```python
from build123d import *

# Parameters (mm, degrees)
BOSS_EXTRUDE1_DEPTH = 10
SKETCH6_W           = 35.294117648
SKETCH6_H           = 18.823529412
BOSS_EXTRUDE3_DEPTH = 500
SKETCH8_W           = 35.294117648
SKETCH8_H           = 20.234009988
BOSS_EXTRUDE4_DEPTH = 50
SKETCH9_W           = 699.8
SKETCH9_H           = 322.2
BOSS_EXTRUDE5_DEPTH = 20
SKETCH10_W          = 689.8
SKETCH10_H          = 302.2
CUT_EXTRUDE1_DEPTH  = 3
CUT_EXTRUDE6_DEPTH  = 5
SKETCH13_W          = 100
SKETCH13_H          = 20
CUT_EXTRUDE7_DEPTH  = 2


with BuildPart() as part:
    # Sketch1 → Boss-Extrude1 (new body)
    with BuildSketch(Plane(origin=(0, 0, 0), x_dir=(1, 0, 0), z_dir=(0, 1, 0))):
        with BuildLine():
            Line((0, 0), (182.11145618, 91.05572809))
            ThreePointArc((182.11145618, 91.05572809), (200, 80), (217.88854382, 91.05572809))
            Line((217.88854382, 91.05572809), (400, 0))
            Line((400, 0), (217.647058824, 109.411764706))
            Line((217.647058824, 109.411764706), (232.214563867, 158.239009858))
            Line((232.214563867, 158.239009858), (200, 120))
            Line((200, 120), (167.785436133, 158.239009858))
            Line((167.785436133, 158.239009858), (182.352941176, 109.411764706))
            Line((182.352941176, 109.411764706), (0, 0))
        make_face()
    extrude(amount=BOSS_EXTRUDE1_DEPTH)

    # Sketch6 → Boss-Extrude3 (add)
    with BuildSketch(Plane(origin=(0, 10, 0), x_dir=(1, 0, 0), z_dir=(0, 1, 0))):
        with Locations((200, 100)):
            Rectangle(SKETCH6_W, SKETCH6_H)
    extrude(amount=BOSS_EXTRUDE3_DEPTH)

    # Sketch8 → Boss-Extrude4 (add)
    with BuildSketch(Plane.XY.offset(-90.588235294)):
        with Locations((200, 346.635085086)):
            Rectangle(SKETCH8_W, SKETCH8_H)
    extrude(amount=BOSS_EXTRUDE4_DEPTH)

    # Sketch9 → Boss-Extrude5 (add)
    with BuildSketch(Plane.XY.offset(-40.588235294)):
        with Locations((200, 346.635085086)):
            Rectangle(SKETCH9_W, SKETCH9_H)
    extrude(amount=BOSS_EXTRUDE5_DEPTH)

    # Sketch10 → Cut-Extrude1 (cut)
    with BuildSketch(Plane.XY.offset(-20.588235294)):
        with Locations((200, 351.635085086)):
            Rectangle(SKETCH10_W, SKETCH10_H)
    extrude(amount=-CUT_EXTRUDE1_DEPTH, mode=Mode.SUBTRACT)

    # Sketch11 → Cut-Extrude6 (cut)
    with BuildSketch(Plane(origin=(0, 0, -40.588235294), x_dir=(-1, 0, 0), z_dir=(0, 0, -1))):
        Polygon((-392.933529412, 226.955085086), (-392.933529412, 225.535085086), (-403.353529412, 225.535085086), (-403.353529412, 226.955085086), (-402.353529412, 227.955085086), (-393.933529412, 227.955085086), align=None)
        Polygon((-366.833529412, 225.535085086), (-366.833529412, 229.295085086), (-367.833529412, 230.295085086), (-382.933529412, 230.295085086), (-382.933529412, 225.535085086), align=None)
        Polygon((-341.733529412, 230.295085086), (-340.733529412, 229.295085086), (-340.733529412, 225.535085086), (-356.833529412, 225.535085086), (-356.833529412, 230.295085086), align=None)
        Polygon((-423.773529412, 226.955085086), (-423.773529412, 225.535085086), (-413.353529412, 225.535085086), (-413.353529412, 226.955085086), (-414.353529412, 227.955085086), (-422.773529412, 227.955085086), align=None)
    extrude(amount=-CUT_EXTRUDE6_DEPTH, mode=Mode.SUBTRACT)

    # Sketch13 → Cut-Extrude7 (cut)
    with BuildSketch(Plane(origin=(0, 0, -40.588235294), x_dir=(-1, 0, 0), z_dir=(0, 0, -1))):
        with Locations((-379.9, 224.097206675)):
            Rectangle(SKETCH13_W, SKETCH13_H)
    extrude(amount=-CUT_EXTRUDE7_DEPTH, mode=Mode.SUBTRACT)


solid = part.part
```
The listing builds one solid part. Answer for the finished solid, in the listing's coordinates (mm). A direction names the side the tool comes from. Coordinates: 2 decimals unless noted, no trailing zeros. Write each loop counter-clockwise with the first axis right and the second up, starting at its lowest first coordinate (ties: lowest second). Pieces come first, ordered by that corner, then holes.
Q1. Section B-B, the plane x = 314.5 is taken. Write down the section's boundary in (y, z), then the cut area to 3 significant figures.
Returned:
outline: (0, -51.3) - (10, -51.3) - (10, -42.75) - (0, -42.75) - close; (185.54, -40.59) - (507.74, -40.59) - (507.74, -20.59) - (502.74, -20.59) - (502.74, -23.59) - (200.54, -23.59) - (200.54, -20.59) - (185.54, -20.59) - close
area: 5,620 mm2
Q2. Section A-A, the plane z = -69 is taken. Write down the section's boundary in (x, y).
Returned:
outline: (115, 0) - (138, 0) - (138, 10) - (115, 10) - close; (182.35, 336.52) - (217.65, 336.52) - (217.65, 356.75) - (182.35, 356.75) - close; (262, 0) - (285, 0) - (285, 10) - (262, 10) - close
Q3. The mould has two halves that part along Z. Classify faces 6 (the flat face through (125, 10, -67)), 7 (the flat face through (174.967, 4.93, -134.167)), 8 (the flat face through (200, 171, -90.588)), 9 (the flat face through (90, 5, -45)): released by +Z, released by -Z, zero draft, split by the parting line, or undercut.
Returned:
face 6: zero draft
face 7: undercut
face 8: undercut
face 9: released by +Z
Q4. Section C-C, the plane y = 475.5 is taken. Write down the section's boundary in (x, z).
Returned:
outline: (-149.9, -40.59) - (549.9, -40.59) - (549.9, -20.59) - (544.9, -20.59) - (544.9, -23.59) - (-144.9, -23.59) - (-144.9, -20.59) - (-149.9, -20.59) - close; (182.35, -109.41) - (217.65, -109.41) - (217.65, -90.59) - (182.35, -90.59) - close
Q5. Find the intervals of material crossed by line 1 along Z through (x, y) = (202, 435); line 2 along Z through (x, y) = (219.5, 230.5); line 3 along Y through (x, z) = (254, -76), in increasing order.
Returned:
line 1: z = -109.41 to -90.59, -40.59 to -23.59
line 2: z = -40.59 to -23.59
line 3: y = 0 to 10
Q6. Given P1, Ø2, axis at x = 390, y = 200.5, coming from the +Z side; P2, Ø10.5, axis at x = 199.5, y = 471, coming from the +Z side; P3, Ø1.5, axis at x = 354, y = 287, coming from the -Z side, each flat-ended and moving along its own axis, determine where each tip first touches the part or whether it passes through.
Returned:
P1: stops at z = -20.59
P2: stops at z = -23.59
P3: stops at z = -40.59
Q7. Which of the six approach directions +Z, -Z, +X, -X, +Y, -Y give full straight-line access (tool end or side, diameter ignored) to faces 1 (the flat face through (200, 256, -109.412)), 2 (the flat face through (224.829, 4.93, -133.484)), 3 (the flat face through (182.353, 259, -95)), 4 (the flat face through (217.647, 259, -95)), 5 (the flat face through (200, 432, -90.588))?
Returned:
face 1: -Z, +X, -X, +Y
face 2: +X, +Y, -Y
face 3: -Z, -X, +Y
face 4: -Z, +X, +Y
face 5: +X, -X, +Y
Q8. Section D-D, the plane x = 457.5 is taken. Write down the section's boundary in (y, z).
Returned:
outline: (185.54, -40.59) - (507.74, -40.59) - (507.74, -20.59) - (502.74, -20.59) - (502.74, -23.59) - (200.54, -23.59) - (200.54, -20.59) - (185.54, -20.59) - close
